Read the model definition and answer for the solid it produces. Units are mm, in the model's axes. A direction names the side the tool comes from. Round coordinates to 2 decimals unless told otherwise and drop trailing zeros. Order: outer loops, then holes, each group sorted by start corner. A loop starts at its lowest first (then second) coordinate and runs counter-clockwise, first axis right, second up.
from build123d import *

# Parameters (mm, degrees)
F0_W     = 44.45
F0_H     = 31.75
F1_DEPTH = 25.4
F2_W     = 44.45
F2_H     = 19.05
F3_DEPTH = 12.7
F5_DEPTH = 25.4
F7_DEPTH = 25.4


with BuildPart() as f1:
    # F0 (on Front) → F1 (new body)
    with BuildSketch(Plane.XZ):
        with Locations((22.225, 15.875)):
            Rectangle(F0_W, F0_H)
    extrude(amount=F1_DEPTH)

    # F2 (on face) → F3 (cut)
    with BuildSketch(Plane.XZ.offset(25.4)):
        with Locations((22.225, 22.225)):
            Rectangle(F2_W, F2_H)
    extrude(amount=-F3_DEPTH, mode=Mode.SUBTRACT)

    # F4 (on face) → F5 (cut)
    with BuildSketch(Plane.XY.offset(12.7)):
        Polygon((44.45, -25.4), (44.45, -12.7), (31.75, -25.4), align=None)
    extrude(amount=-F5_DEPTH, mode=Mode.SUBTRACT)

    # F6 (on face) → F7 (cut)
    with BuildSketch(Plane.XZ.offset(12.7)):
        Polygon((31.75, 31.75), (44.45, 12.7), (44.45, 31.75), align=None)
    extrude(amount=-F7_DEPTH, mode=Mode.SUBTRACT)


solid = f1.part
Q1. For faces 1 (the face through (17, -19, 12.7)), 2 (the face through (16, -6, 31.75)), determine the directions among +Z, -Z, +X, -X, +Y, -Y from which every point of the face is accessible in a straight line to the end or side of a thin tool.
Outcome:
face 1: +Z, +X, -X, -Y
face 2: +Z, +X, -X, +Y, -Y
Q2. Straight lines are drawn through the part: probe 1 along Z at (x, y) = (9, -21.25); probe 2 along Y at (x, z) = (16, 17); probe 3 along X at (y, z) = (-5.25, 19.5). For each, find the intervals that lie inside material, in ascending order.
Outcome:
probe 1: z = 0 to 12.7
probe 2: y = -12.7 to 0
probe 3: x = 0 to 39.92
Q3. A cutting plane is placed at D-D, the plane x = 38.5. Give the vertices of the cut face in (y, z) (3 decimals), plus the area to 3 significant figures.
Outcome:
outline: (-18.65, 0) - (0, 0) - (0, 21.625) - (-12.7, 21.625) - (-12.7, 12.7) - (-18.65, 12.7) - close
area: 350 mm2
Q4. A cutting plane is placed at A-A, the plane x = 12. Give the vertices of the cut face in (y, z).
Outcome:
outline: (-25.4, 0) - (0, 0) - (0, 31.75) - (-12.7, 31.75) - (-12.7, 12.7) - (-25.4, 12.7) - close
Q5. A cutting plane is placed at C-C, the plane y = -16. Give the vertices of the cut face in (x, z).
Outcome:
outline: (0, 0) - (41.15, 0) - (41.15, 12.7) - (0, 12.7) - close
Q6. Flat-ended cylindrical pins translate along their axes: pin 1 (5 mm diameter, centred on x = 38.5, y = -9, fed in from +Z) (3 decimals); pin 2 (1.5 mm diameter, centred on x = 38, z = 14, fed in from -Y); pin 3 (4 mm diameter, centred on x = 25, y = -17, fed in from +Z). Find the tip coordinate at first contact, or state that the pin passes through.
Outcome:
pin 1: stops at z = 25.375
pin 2: stops at y = -12.7
pin 3: stops at z = 12.7
Q7. A cutting plane is placed at B-B, the plane z = 8. Give the vertices of the cut face in (x, y), plus the area to 3 significant figures.
Outcome:
outline: (0, -25.4) - (31.75, -25.4) - (44.45, -12.7) - (44.45, 0) - (0, 0) - close
area: 1,050 mm2
